The model under review builds one solid part; all positions refer to its coordinate system, in mm. A direction names the side the tool comes from. Coordinates: 2 decimals unless noted, no trailing zeros. Order: outer loops, then holes, each group sorted by start corner. A loop starts at its lowest first (then second) coordinate and runs counter-clockwise, first axis right, second up. Notation, with made-up numbers: M 33,51.5 L 58,51.5 A16 cw 58,64.5 Z; hole C 31.25,41.25 d4. An arc over 180 degrees is marked long. One line per item, written item: value.
```python
from build123d import *

# Parameters (mm, degrees)
F0_W     = 382
F0_H     = 18
F0_W_2   = 700
F0_H_2   = 630
F0_W_3   = 664
F0_H_3   = 594
F0_H_4   = 315
F0_H_5   = 279
F0_W_4   = 50
F1_DEPTH = 600
F2_W     = 2670
F2_H     = 630
F3_DEPTH = 18


with BuildPart() as f1:
    # F0 (on Front) → F1 (new body)
    with BuildSketch(Plane.XZ):
        with Locations((209, 9)):
            Rectangle(F0_W, F0_H)
        Polygon((0, 630), (0, 0), (18, 0), (18, 18), (18, 182), (18, 200), (18, 400), (18, 418), (18, 612), (400, 612), (400, 418), (400, 400), (400, 200), (400, 182), (400, 18), (400, 0), (440, 0), (440, 630), (400, 630), align=None)
        with Locations((790, 315)):
            Rectangle(F0_W_2, F0_H_2)
        with Locations((790, 315)):
            Rectangle(F0_W_3, F0_H_3, mode=Mode.SUBTRACT)
        Polygon((1140, 630), (1140, 0), (1180, 0), (1180, 315), (1180, 630), align=None)
        with Locations((1530, 472.5)):
            Rectangle(F0_W_2, F0_H_4)
        with Locations((1530, 472.5)):
            Rectangle(F0_W_3, F0_H_5, mode=Mode.SUBTRACT)
        with Locations((1530, 157.5)):
            Rectangle(F0_W_2, F0_H_4)
        Polygon((1198, 297), (1862, 297), (1862, 156), (1862, 138), (1862, 18), (1198, 18), (1198, 138), (1198, 156), align=None, mode=Mode.SUBTRACT)
        Polygon((1880, 315), (1880, 0), (1920, 0), (1920, 315), (1920, 630), (1880, 630), align=None)
        Polygon((1920, 315), (1920, 0), (2620, 0), (2620, 630), (1920, 630), align=None)
        with Locations((2270, 315)):
            Rectangle(F0_W_3, F0_H_3, mode=Mode.SUBTRACT)
        with Locations((2645, 315)):
            Rectangle(F0_W_4, F0_H_2)
        with Locations((209, 191)):
            Rectangle(F0_W, F0_H)
        with Locations((209, 409)):
            Rectangle(F0_W, F0_H)
        with Locations((1530, 147)):
            Rectangle(F0_W_3, F0_H)
    extrude(amount=-F1_DEPTH)

    # F2 (on face) → F3 (join)
    with BuildSketch(Plane(origin=(0, 600, 0), x_dir=(-1, 0, 0), z_dir=(0, 1, 0))):
        with Locations((-1335, 315)):
            Rectangle(F2_W, F2_H)
    extrude(amount=-F3_DEPTH)


solid = f1.part
```
(1) We need section B-B, the plane z = 87.5. State the section outline as (x, y) points.
Geometry results:
outline: M 0,0 L 18,0 L 18,582 L 400,582 L 400,0 L 458,0 L 458,582 L 1122,582 L 1122,0 L 1198,0 L 1198,582 L 1862,582 L 1862,0 L 1938,0 L 1938,582 L 2602,582 L 2602,0 L 2670,0 L 2670,600 L 0,600 Z
(2) Mouldability with a two-part tool opening along X and no side actions: class faces 3 (the flat face through (2602, 287, 311)), 4 (the flat face through (1316, 600, 319)) as +X half, -X half, draft (parallel to the pull), parting line (faces both ways), or undercut.
Geometry results:
face 3: undercut
face 4: draft
(3) For L1, parallel to X at y = 271, z = 306.5; L2, parallel to X at y = 400.5, z = 427; L3, parallel to Z at x = 1716.5, y = 370, list the stretches that pass through material, from the lowest coordinate up.
Geometry results:
L1: x = 0 to 18, 400 to 458, 1122 to 1938, 2602 to 2670
L2: x = 0 to 18, 400 to 458, 1122 to 1198, 1862 to 1938, 2602 to 2670
L3: z = 0 to 18, 138 to 156, 297 to 333, 612 to 630
(4) Tool access review of faces 1 (the flat face through (458, 287, 311)), 2 (the flat face through (1428, 0, 316)): name each direction out of +Z, -Z, +X, -X, +Y, -Y from which nothing blocks a thin tool from reaching the whole face with its end or side.
Geometry results:
face 1: -Y
face 2: +Z, -Z, +X, -X, -Y
(5) Insertion check: pin 1 Ø5 at (x, z) = (1339.5, 101.5) entering from -Y. The pin has a flat end and moves straight along its axis. Give the tip position at first contact, or say it passes through.
Geometry results:
pin 1: stops at y = 582
(6) We need section A-A, the plane x = 1290. State the section outline as (y, z) points, plus the area to 3 significant figures.
Geometry results:
outline: M 0,0 L 600,0 L 600,630 L 0,630 L 0,612 L 582,612 L 582,333 L 0,333 L 0,297 L 582,297 L 582,156 L 0,156 L 0,138 L 582,138 L 582,18 L 0,18 Z
area: 63,700 mm2
(7) We need section D-D, the plane x = 2375.5. State the section outline as (y, z) points, plus the area to 3 significant figures.
Geometry results:
outline: M 0,0 L 600,0 L 600,630 L 0,630 L 0,612 L 582,612 L 582,18 L 0,18 Z
area: 32,300 mm2
(8) We need section C-C, the plane y = 360. Count the separate pieces of the cut face and the enclosed holes in it, plus the area to 3 significant figures.
Geometry results:
separate pieces: 1
enclosed holes: 8
area: 322,000 mm2
